from build123d import *

# Parameters (mm, degrees)
F0_R      = 19.265609
F1_DEPTH  = 28.194
F2_R      = 76.715917
F3_DEPTH  = 9.652
F4_SIZE   = 10.16
F5_R      = 76.623003
F5_R_2    = 65.62423
F6_DEPTH  = 17.78
F7_R      = 140.410315
F7_R_2    = 73.406881
F8_DEPTH  = 65.024
F9_R      = 22.075569
F10_R     = 7.246606
F10_R_2   = 6.662483
F10_R_3   = 6.800081
F10_R_4   = 5.519125
F11_DEPTH = 37.846
F12_R     = 12.893093
F13_DEPTH = 170.434
F14_W     = 70.021615
F14_H     = 44.968011
F15_DEPTH = 22.352
F16_W     = 27.50209
F16_H     = 304.814771
F17_DEPTH = 12.7


with BuildPart() as f1:
    # F0 (on Front) → F1 (new body, symmetric)
    with BuildSketch(Plane.XZ):
        Circle(F0_R)
    extrude(amount=F1_DEPTH, both=True)

    # F2 (on Front) → F3 (join, symmetric)
    with BuildSketch(Plane.XZ):
        Circle(F2_R)
    extrude(amount=F3_DEPTH, both=True)

    # F4
    f4_edges = [f1.edges().sort_by_distance(p)[0] for p in [
        (-19.265609, -28.194, 0),
    ]]
    chamfer(f4_edges, length=F4_SIZE)

    # F5 (on Front) → F6 (join, symmetric)
    with BuildSketch(Plane.XZ):
        Circle(F5_R)
        Circle(F5_R_2, mode=Mode.SUBTRACT)
    extrude(amount=F6_DEPTH, both=True)

    # F7 (on Front) → F8 (join, symmetric)
    with BuildSketch(Plane.XZ):
        Circle(F7_R)
        Circle(F7_R_2, mode=Mode.SUBTRACT)
    extrude(amount=F8_DEPTH, both=True)

    # F9
    f9_edges = [f1.edges().sort_by_distance(p)[0] for p in [
        (-140.410315, 65.024, 0),
        (-73.406881, 65.024, 0),
        (-140.410315, -65.024, 0),
        (-73.406881, -65.024, 0),
    ]]
    fillet(f9_edges, radius=F9_R)

    # F10 (on Front) → F11 (join, symmetric)
    with BuildSketch(Plane.XZ):
        with Locations((0, 43.201409)):
            Circle(F10_R)
        with Locations((41.43481, 0)):
            Circle(F10_R_2)
        with Locations((0, -41.274209)):
            Circle(F10_R_3)
        with Locations((-39.507613, 0)):
            Circle(F10_R_4)
    extrude(amount=F11_DEPTH, both=True)

    # F12 (on Front) → F13 (join)
    with BuildSketch(Plane.XZ):
        Circle(F12_R)
    extrude(amount=-F13_DEPTH)

    # F14 (on Right) → F15 (join, symmetric)
    with BuildSketch(Plane.YZ):
        with Locations((145.725421, 0.803)):
            Rectangle(F14_W, F14_H)
    extrude(amount=F15_DEPTH, both=True)

    # F16 (on Right) → F17 (join, symmetric)
    with BuildSketch(Plane.YZ):
        with Locations((146.83339, 163.384787)):
            Rectangle(F16_W, F16_H)
    extrude(amount=F17_DEPTH, both=True)


solid = f1.part
The listing builds one solid part. Answer for the finished solid, in the listing's coordinates (mm). A direction names the side the tool comes from. Round coordinates to 2 decimals unless told otherwise and drop trailing zeros. Write each loop counter-clockwise with the first axis right and the second up, starting at its lowest first coordinate (ties: lowest second). Pieces come first, ordered by that corner, then holes. Notation, with made-up numbers: (-3.75, 55.5) - (44.25, 55.5) arc R28 ccw to (44.25, 75.5) - close; hole circle Ø1 at (68, -40). An arc over 180 degrees is marked (long way). Use one line per item in the form item = value. Start each with the question number.
Item 1: Find the intervals of material crossed by line 1 (Z direction, x = 0, y = -33); line 2 (Z direction, x = 0, y = -14); line 3 (Y direction, x = -53, z = 84.5), in increasing order. Write a range as [from, to].
Item 2: A cutting plane is placed at B-B (z = 224.5). Write down the section's boundary in (x, y), plus the area to 3 significant figures.
Item 3: Determine the mould class of faces 1 (the cylindrical face through (133.926, -0.601, 42.175)), 2 (the cylindrical face through (-0.943, 23.552, 50.386)), 3 (the flat face through (0, 133.082, 167)) for opening direction Z: +Z half, -Z half, draft (parallel to the pull), parting line (faces both ways), or undercut.
Item 4: Flat-ended cylindrical pins translate along their axes: pin 1 Ø10.5 at (x, z) = (41.5, -2.5) entering from -Y; pin 2 Ø10 at (x, z) = (7, 220.5) entering from +Y; pin 3 Ø1 at (x, y) = (63.5, -26.5) entering from -Z; pin 4 Ø10 at (y, z) = (126.5, 133) entering from +X. Find the tip coordinate at first contact, or state that the pin passes through.
Item 5: A tool of negligible diameter and unlimited length cuts with its end or side. For faces 4 (the flat face through (-40, 37.846, 0)), 5 (the flat face through (0, -37.846, -41)), 6 (the flat face through (0, 37.846, 43)), from which of +Z, -Z, +X, -X, +Y, -Y can it reach the whole face along a straight path? Write none if from no direction.
Item 6: A cutting plane is placed at A-A (y = 104). Write down the section's boundary in (x, z), plus the area to 3 significant figures.
The answers:
q1.line_1 = [-140.41, -73.41], [-48.07, -34.47], [35.95, 50.45], [73.41, 140.41]
q1.line_2 = [-140.41, -65.62], [-48.07, -34.47], [-19.27, 19.27], [35.95, 50.45], [65.62, 140.41]
q1.line_3 = [-65.02, 65.02]
q2.outline = (-12.7, 133.08) - (12.7, 133.08) - (12.7, 160.58) - (-12.7, 160.58) - close
q2.area = 699 mm^2
q3.face_1 = parting line
q3.face_2 = undercut
q3.face_3 = draft
q4.pin_1 = -37.85
q4.pin_2 = 160.58
q4.pin_3 = -125.48
q4.pin_4 = through
q5.face_4 = +Y
q5.face_5 = -Y
q5.face_6 = none
q6.outline = circle Ø25.79 at (0, 0)
q6.area = 522 mm^2
